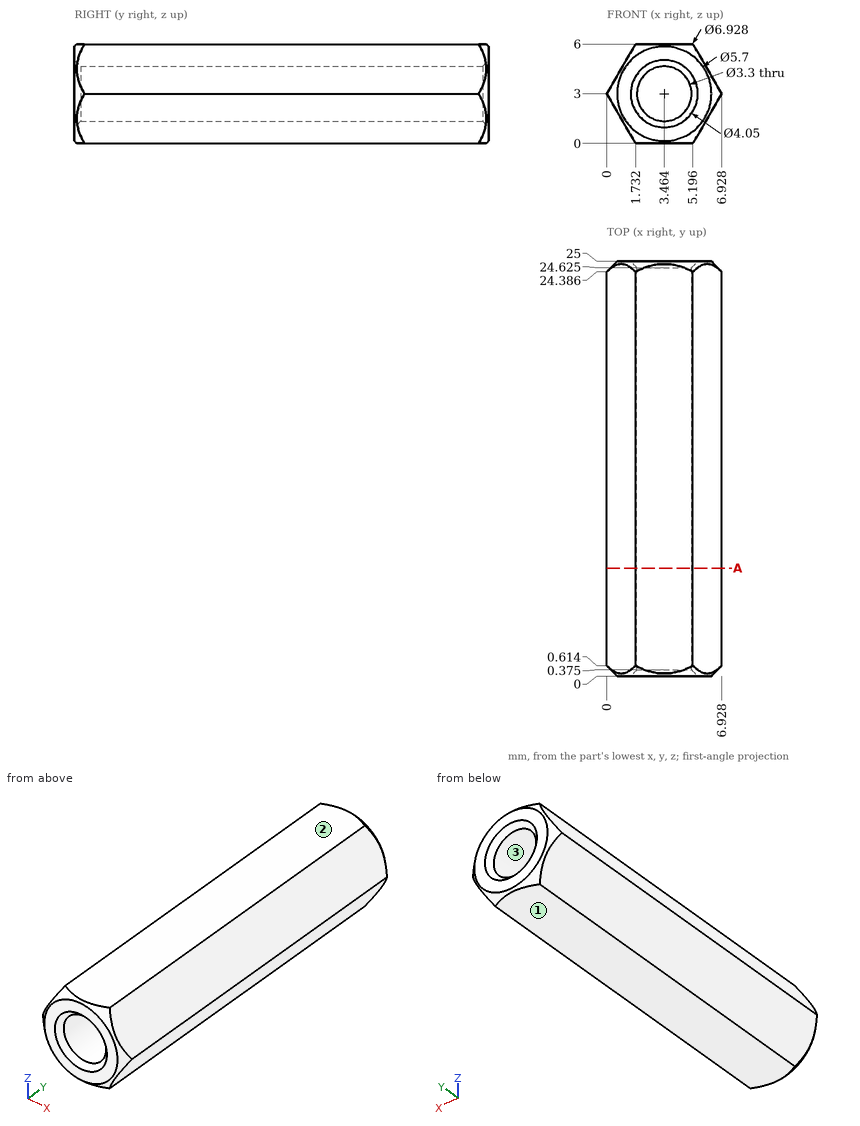
Part print with two shaded views. Sizes in mm from the minimum x, y, z corner. Coordinates: 2 decimals unless noted, no trailing zeros. Write each loop counter-clockwise with the first axis right and the second up, starting at its lowest first coordinate (ties: lowest second). Pieces come first, ordered by that corner, then holes. Notation, with made-up numbers: M -36,15 L 17,15 A31 ccw 17,46 Z; hole C 20,28 d3. An arc over 180 degrees is marked long. Return JSON: item names as keys, results as strings.
Item 1: Probe line 1 (Z direction, x = 3.5, y = 11); line 2 (Z direction, x = 2, y = 8); line 3 (X direction, y = 21.25, z = 2.6) (1 decimal). List the from-to ranges inside material, lowest first. Write a range as from..to.
Findings below:
{"line 1": "z = 0..1.35, 4.65..6", "line 2": "z = 0..2.24, 3.76..6", "line 3": "x = 0.2..1.9, 5.1..6.7"}
Item 2: Slice it at A-A, the plane y = 6.5. Write the cut outline in (x, z).
Findings below:
{"outline": "M 0,3 L 1.73,0 L 5.2,0 L 6.93,3 L 5.2,6 L 1.73,6 Z; hole C 3.46,3 d3.3"}
Item 3: Drop a flat-ended pin along its axis: pin 1 Ø3 at (y, z) = (9, 5) entering from +X. Give the stop position or say it passes through.
Findings below:
{"pin 1": "stops at x = 6.64"}
Item 4: Two-plate mould, pull along Z, no slides. Class the marked faces 1, 2 and 3: +Z half, -Z half, draft (parallel to the pull), parting line (faces both ways), or undercut.
Findings below:
{"face 1": "-Z half", "face 2": "+Z half", "face 3": "undercut"}
